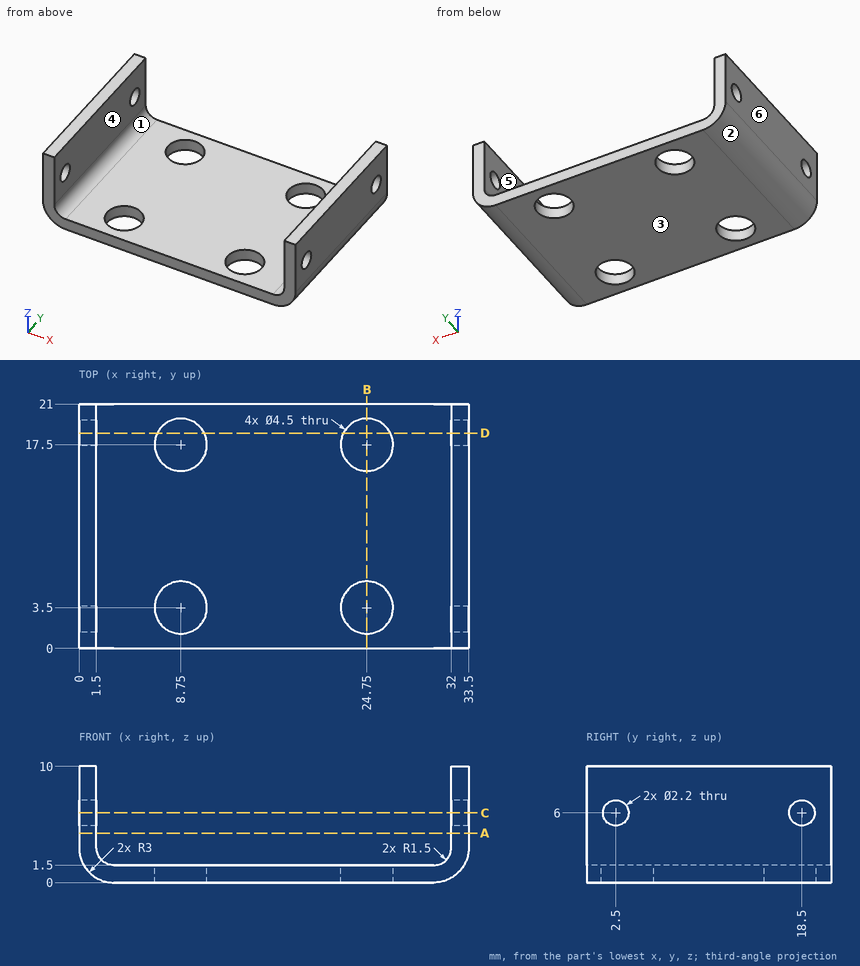
Could you check a few things on this drawing? It's one solid part, dimensions in mm from its lowest x, y, z. A direction names the side the tool comes from. Coordinates: 2 decimals unless noted, no trailing zeros. Write each loop counter-clockwise with the first axis right and the second up, starting at its lowest first coordinate (ties: lowest second). Pieces come first, ordered by that corner, then holes. Notation, with made-up numbers: (29, -39.75) - (80, -39.75) arc R29 ccw to (80, -18.75) - close; hole circle Ø3 at (-40, -29.5). An arc over 180 degrees is marked (long way). Write item = value, one per line.
1) Suppose I cut it at C-C on z = 6. Please give me the cut outline in (x, y), plus the area to 3 significant figures.
Result set:
outline = (0, 0) - (1.5, 0) - (1.5, 1.4) - (0, 1.4) - close; (0, 3.6) - (1.5, 3.6) - (1.5, 17.4) - (0, 17.4) - close; (0, 19.6) - (1.5, 19.6) - (1.5, 21) - (0, 21) - close; (32, 0) - (33.5, 0) - (33.5, 1.4) - (32, 1.4) - close; (32, 3.6) - (33.5, 3.6) - (33.5, 17.4) - (32, 17.4) - close; (32, 19.6) - (33.5, 19.6) - (33.5, 21) - (32, 21) - close
area = 49.8 mm2
2) For the marked faces 5 and 6, which set-ups out of +Z, -Z, +X, -X, +Y, -Y let a thin tool reach every point of the face, with its end or its side?
Result set:
face_5 = +Z, +Y, -Y
face_6 = +Z, -Z, -X, +Y, -Y
3) Will these pins go through, and if not, where does the flat tip stop? pin 1 Ø2 at (x, y) = (19, 8.5) entering from +Z; pin 2 Ø1.8 at (y, z) = (2.5, 6) entering from -X.
Result set:
pin_1 = 1.5
pin_2 = through
4) Suppose I cut it at A-A on z = 4.25. Please give me the cut outline in (x, y), plus the area to 3 significant figures.
Result set:
outline = (0, 0) - (1.5, 0) - (1.5, 21) - (0, 21) - close; (32, 0) - (33.5, 0) - (33.5, 21) - (32, 21) - close
area = 63.0 mm2
5) Suppose I cut it at D-D on y = 18.5. Please give me the cut outline in (x, z), plus the area to 3 significant figures.
Result set:
outline = (0, 3) arc R3 ccw to (3, 0) - (6.73, 0) - (6.73, 1.5) - (3, 1.5) arc R1.5 cw to (1.5, 3) - (1.5, 4.9) - (0, 4.9) - close; (0, 7.1) - (1.5, 7.1) - (1.5, 10) - (0, 10) - close; (10.77, 0) - (22.73, 0) - (22.73, 1.5) - (10.77, 1.5) - close; (26.77, 0) - (30.5, 0) arc R3 ccw to (33.5, 3) - (33.5, 4.9) - (32, 4.9) - (32, 3) arc R1.5 cw to (30.5, 1.5) - (26.77, 1.5) - close; (32, 7.1) - (33.5, 7.1) - (33.5, 10) - (32, 10) - close
area = 54.2 mm2
6) Please list where these lines run through material, in increasing order: line 1 (Y direction, x = 32.4, z = 6); line 2 (Y direction, x = 24.75, z = 0.6); line 3 (X direction, y = 3.5, z = 0.4). Write a range as [from, to].
Result set:
line_1 = [0, 1.4], [3.6, 17.4], [19.6, 21]
line_2 = [0, 1.25], [5.75, 15.25], [19.75, 21]
line_3 = [1.5, 6.5], [11, 22.5], [27, 32]
7) Suppose I cut it at B-B on x = 24.75. Please give me the cut outline in (y, z), plus the area to 3 significant figures.
Result set:
outline = (0, 0) - (1.25, 0) - (1.25, 1.5) - (0, 1.5) - close; (5.75, 0) - (15.25, 0) - (15.25, 1.5) - (5.75, 1.5) - close; (19.75, 0) - (21, 0) - (21, 1.5) - (19.75, 1.5) - close
area = 18.0 mm2
8) We'd pull the mould along X, two halves only. Please class the marked faces 1, 2, 3 and 4: +X half, -X half, draft (parallel to the pull), parting line (faces both ways), or undercut.
Result set:
face_1 = undercut
face_2 = -X half
face_3 = draft
face_4 = undercut
